Autodesk Inventor part; units mm, degrees
ref_plane "YZ Plane" through (0, 0, 0) normal (1, 0, 0) x (0, 1, 0)
ref_plane "XZ Plane" through (0, 0, 0) normal (0, 1, 0) x (-1, 0, 0)
ref_plane "XY Plane" through (0, 0, 0) normal (0, 0, 1) x (1, 0, 0)
sketch "Sketch1" plane through (0, 0, 0) normal (0, 0, 1) x (1, 0, 0)
  line L0 (-12.0255, 5.2117) -> (16.8797, 5.2117)
  line L1 (16.8797, 5.2117) -> (16.8797, -7.7423)
  line L2 (16.8797, -7.7423) -> (-12.0255, -7.7423)
  line L3 (-12.0255, -7.7423) -> (-12.0255, 5.2117)
  point P0 (0, 0)
  dimension "d0" = 12.954
  dimension "d1" = 28.9052
extrude "Extrusion1" add sketch "Sketch1" along normal blind 18.3388
sketch "Sketch2" plane through (-12.0255, 5.2117, 0) normal (0, 1, 0) x (1, 0, 0)
  line L0 (0, 0) -> (28.9052, 0)
  line L1 (28.9052, -18.3388) -> (0, -18.3388)
  line L2 (0, 0) -> (0, -18.3388)
  circle A0 centre (14.4526, -9.1694) radius 5.8547
  point P0 (12.0255, 0)
  dimension "d4" = 11.7094
extrude "Extrusion2" add sketch "Sketch2" along normal blind 9.3472
sketch "Sketch3" plane through (2.4271, 14.5589, 9.1694) normal (0, 1, 0) x (1, 0, 0)
  circle A0 centre (0, 0) radius 3.0988
  point P0 (-2.4271, 9.1694)
  dimension "d7" = 6.1976
extrude "Extrusion3" cut sketch "Sketch3" against normal blind 1.27
sketch "Sketch4" plane through (2.4271, 13.2889, 9.1694) normal (0, 1, 0) x (1, 0, 0)
  circle A0 centre (0, 0) radius 2.2352
  point P0 (-2.4271, 9.1694)
  dimension "d10" = 4.4704
extrude "Extrusion4" add sketch "Sketch4" along normal blind 19.0754
properties part number "mcdave_switch"
Could you check a few things on this model? Use its own coordinates, in mm. A direction names the side the tool comes from. Round coordinates to 2 decimals unless told otherwise and drop trailing zeros. Loops run counter-clockwise (first coordinate to the right, second up) from the corner with the lowest first, then second, coordinate; pieces in that order, holes last. Notation, with made-up numbers: (-38.5, 13.25) -> (12.5, 13.25) arc R10 ccw to (12.5, 32.25) -> close; hole circle Ø6 at (80, 11). An arc over 180 degrees is marked (long way). Use CSV: the item, a comma, the result in double quotes.
(1) Suppose I cut it at D-D on z = 2. Write out the boundary of the cut face in (x, y).
Return value:
outline,"(-12.03, -7.74) -> (16.88, -7.74) -> (16.88, 5.21) -> (-12.03, 5.21) -> close"
(2) For faces 1 (the flat face through (5, 14.559, 12)), 2 (the flat face through (2, 32.364, 9)), which set-ups out of +Z, -Z, +X, -X, +Y, -Y let a thin tool reach every point of the face, with its end or its side?
Return value:
face 1,"+Y"
face 2,"+Z, -Z, +X, -X, +Y"
(3) If I drill on probe 1 along X at (y, z) = (14, 11); probe 2 along Y at (x, z) = (-6.25, 12); probe 3 along Y at (x, z) = (2.5, 4.75), over which ranges is the centre line in solid material (lowest first)? Write a range as [from, to].
Return value:
probe 1,"x = [-3.13, -0.07], [1.14, 3.71], [4.93, 7.99]"
probe 2,"y = [-7.74, 5.21]"
probe 3,"y = [-7.74, 14.56]"
(4) Suppose I cut it at A-A on z = 7.5. Write out the boundary of the cut face in (x, y).
Return value:
outline,"(-12.03, -7.74) -> (16.88, -7.74) -> (16.88, 5.21) -> (8.04, 5.21) -> (8.04, 14.56) -> (5.04, 14.56) -> (5.04, 13.29) -> (3.91, 13.29) -> (3.91, 32.36) -> (0.94, 32.36) -> (0.94, 13.29) -> (-0.18, 13.29) -> (-0.18, 14.56) -> (-3.18, 14.56) -> (-3.18, 5.21) -> (-12.03, 5.21) -> close"
(5) Suppose I cut it at C-C on y = 14. Write out the boundary of the cut face in (x, z).
Return value:
outline,"circle Ø11.71 at (2.43, 9.17); circle Ø4.47 at (2.43, 9.17); hole circle Ø6.2 at (2.43, 9.17)"
(6) Suppose I cut it at B-B on x = -8. Write out the boundary of the cut face in (y, z), plus the area to 3 significant figures.
Return value:
outline,"(-7.74, 0) -> (5.21, 0) -> (5.21, 18.34) -> (-7.74, 18.34) -> close"
area,"238 mm²"
(7) If we mould it in two halves opening along Z, with no side actions, what happens to faces 3 (the flat face through (2, 5.212, 3)), 4 (the flat face through (2, -1, 0)), 5 (the flat face through (1, 13.289, 7)), 6 (the flat face through (2, -1, 18.339))? For each: +Z half, -Z half, draft (parallel to the pull), parting line (faces both ways), or undercut.
Return value:
face 3,"draft"
face 4,"-Z half"
face 5,"undercut"
face 6,"+Z half"
(8) Will these pins go through, and if not, where does the flat tip stop? pin 1 Ø6 at (x, z) = (10.5, 11.5) entering from +Y; pin 2 Ø6 at (x, y) = (5.5, 18) entering from +Z; pin 3 Ø5 at (x, y) = (-2.5, 16.5) entering from -Z.
Return value:
pin 1,"stops at y = 14.56"
pin 2,"stops at z = 11.4"
pin 3,"stops at z = 4.37"
